Model file for the job. Use its own axes, mm. Face numbers are marked on the shaded views. A direction names the side the tool comes from. Give positions to 0.01 mm unless a question says otherwise; leave off trailing zeros. Loops run counter-clockwise (first coordinate to the right, second up) from the corner with the lowest first, then second, coordinate; pieces in that order, holes last. Notation, with made-up numbers: M 86,11.25 L 132,11.25 A23 ccw 132,34.25 Z; hole C 7.25,7 d11. An arc over 180 degrees is marked long. Use CSV: the item, a comma, the result in double quotes. Start each with the question number.
(1) Slice it at C-C on y = 12. List the corners of the cut face in (x, z), and give its area (3 significant figures).
(2) Slice it at D-D on x = 11.5. List the corners of the cut face in (y, z), and give its area (3 significant figures).
(3) Flat gauge pins, fed straight in: P1, Ø12, axis at x = 29.5, z = 12.5, coming from the +Y side; P2, Ø20, axis at x = 36.5, y = 12, coming from the -Z side; P3, Ø10, axis at x = 28, y = 16.5, coming from the +Z side. Where does each tip first touch, or does it go through?
(4) Two-plate mould, pull along Z, no slides. Class the marked faces 4, 5, 6 and 7: pulls with the +Z half, pulls with the -Z half, needs draft (parallel to the pull), parting line crosses it, or undercut.
(5) Slice it at A-A on x = 30. List the corners of the cut face in (y, z).
(6) Wall check: line 1 along X through (y, z) = (1, 0); line 2 along X through (y, z) = (22.5, 22); line 3 along Y through (x, z) = (20, 20). Give the ranges that are in metal, low to high. Write a range as from..to.
(7) Slice it at B-B on z = 0. List the corners of the cut face in (x, y).
(8) Tool access for the marked faces 1, 2 and 3: list every direction of +Z, -Z, +X, -X, +Y, -Y with a clear straight run to the whole face (end or side of a thin tool).
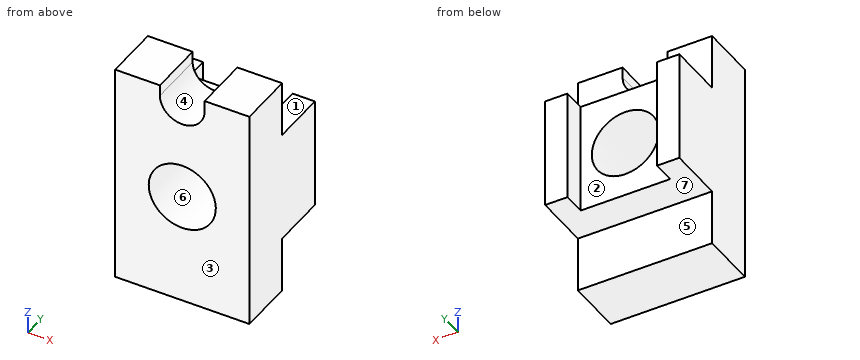
```python
from build123d import *

# Parameters (mm, degrees)
BOSS_EXTRU_1_DEPTH      = 60
ENL_V_MAT_EXTRU_1_DEPTH = 83.006097334
ESQUISSE3_W             = 40
ESQUISSE3_H             = 50
ENL_V_MAT_EXTRU_2_DEPTH = 10
ESQUISSE4_R             = 15
ENL_V_MAT_EXTRU_3_DEPTH = 88.749643874


with BuildPart() as part:
    # Esquisse1 → Boss.-Extru.1 (new body)
    with BuildSketch(Plane(origin=(0, 0, 0), x_dir=(0, 0, -1), z_dir=(1, 0, 0))):
        Polygon((-50, 0), (-25, 0), (-25, 25), (25, 25), (25, 0), (50, 0), (50, -25), (-50, -25), align=None)
    extrude(amount=BOSS_EXTRU_1_DEPTH)

    # Esquisse2 → Enlèv. mat.-Extru.1 (cut, through all)
    with BuildSketch(Plane(origin=(0, 0, 0), x_dir=(1, 0, 0), z_dir=(0, 1, 0))):
        with BuildLine():
            Line((40, -45), (40, -60))
            ThreePointArc((40, -60), (30, -70), (20, -60))
            Line((20, -60), (20, -45))
            ThreePointArc((20, -45), (30, -35), (40, -45))
        make_face()
    extrude(amount=-ENL_V_MAT_EXTRU_1_DEPTH, mode=Mode.SUBTRACT)

    # Esquisse3 → Enlèv. mat.-Extru.2 (cut)
    with BuildSketch(Plane(origin=(0, 25, 0), x_dir=(1, 0, 0), z_dir=(0, 1, 0))):
        with Locations((30, 0)):
            Rectangle(ESQUISSE3_W, ESQUISSE3_H)
    extrude(amount=-ENL_V_MAT_EXTRU_2_DEPTH, mode=Mode.SUBTRACT)

    # Esquisse4 → Enlèv. mat.-Extru.3 (cut, through all)
    with BuildSketch(Plane(origin=(0, 15, 0), x_dir=(1, 0, 0), z_dir=(0, 1, 0))):
        with Locations(Location((30, 0, 0), (0, 0, 270))):
            Circle(ESQUISSE4_R)
    extrude(amount=-ENL_V_MAT_EXTRU_3_DEPTH, mode=Mode.SUBTRACT)


solid = part.part
```
Reply:
1,outline,"M 0,-25 L 60,-25 L 60,25 L 0,25 Z; hole C 30,0 d30"
1,area,"2,290 mm^2"
2,outline,"M -25,-50 L 0,-50 L 0,-25 L 15,-25 L 15,25 L 0,25 L 0,50 L -25,50 Z"
2,area,"3,250 mm^2"
3,P1,"stops at y = 15"
3,P2,"stops at z = -25"
3,P3,"stops at z = 25"
4,face 4,"pulls with the +Z half"
4,face 5,"needs draft"
4,face 6,"undercut"
4,face 7,"pulls with the -Z half"
5,outline,"M -25,-50 L 0,-50 L 0,-25 L 15,-25 L 15,-15 L -25,-15 Z; M -25,15 L 15,15 L 15,25 L 0,25 L 0,35 L -25,35 Z"
6,line 1,"x = 0..15, 45..60"
6,line 2,"x = 0..10, 50..60"
6,line 3,"y = -25..15"
7,outline,"M 0,-25 L 15,-25 L 15,15 L 10,15 L 10,25 L 0,25 Z; M 45,-25 L 60,-25 L 60,25 L 50,25 L 50,15 L 45,15 Z"
8,face 1,"+Z, +X, -X, +Y"
8,face 2,"+Z, -Z, +Y"
8,face 3,"+Z, -Z, +X, -X, -Y"
